from build123d import *

# Parameters (mm, degrees)
BOSS_EXTRUDE1_DEPTH = 50
BOSS_EXTRUDE2_DEPTH = 140.997088


with BuildPart() as part:
    # Sketch2 → Boss-Extrude1 (new body)
    with BuildSketch(Plane.XY.offset(17)):
        with BuildLine():
            Line((70.444464788, 96.391350971), (18.723576719, 85.49867955))
            ThreePointArc((18.723576719, 85.49867955), (18.658589867, 95.297259441), (14.88570491, 86.253934263))
            Line((14.88570491, 86.253934263), (-14.993863644, 86.253934263))
            ThreePointArc((-14.993863644, 86.253934263), (-18.766748601, 95.297259441), (-18.831735453, 85.49867955))
            Line((-18.831735453, 85.49867955), (-70.552623522, 96.391350971))
            Line((-70.552623522, 96.391350971), (-70.552623522, 101.391350971))
            Line((-70.552623522, 101.391350971), (70.444464788, 101.391350971))
            Line((70.444464788, 101.391350971), (70.444464788, 96.391350971))
        make_face()
    extrude(amount=-BOSS_EXTRUDE1_DEPTH)

    # Sketch7 → Boss-Extrude2 (add)
    with BuildSketch(Plane.ZY.offset(70.552623522)):
        Polygon((17, 131.391350971), (2, 131.391350971), (-33, 101.391350971), (17, 101.391350971), align=None)
    extrude(amount=-BOSS_EXTRUDE2_DEPTH)


solid = part.part
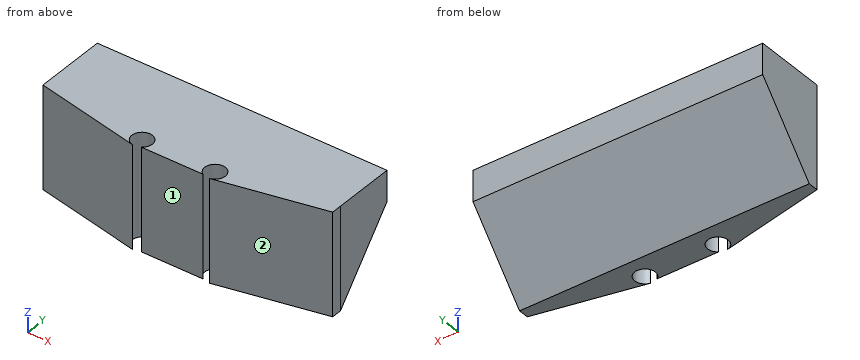
CAD build for the part. Positions are in the model's coordinates, mm. Face numbers are marked on the shaded views. A direction names the side the tool comes from. Round coordinates to 2 decimals unless told otherwise and drop trailing zeros. Loops run counter-clockwise (first coordinate to the right, second up) from the corner with the lowest first, then second, coordinate; pieces in that order, holes last.
(1) Which spindle directions (+Z, -Z, +X, -X, +Y, -Y) get a long thin tool onto all of the face, cutting with end or side? Do the marked faces 1 and 2. Say none if no direction does.
(2) Cut at A-A (y = 92.5). Give the cut face in (x, z).
(3) Cut at B-B (x = 0.5). Give the cut face in (y, z), plus the area to 3 significant figures.
(4) Cut at C-C (z = -16). Give the cut face in (x, y), plus the area to 3 significant figures.
(5) Drop flat-ended pins along their axis: pin 1 (4 mm diameter, centred on x = -9, z = -7, fed in from +Y); pin 2 (2 mm diameter, centred on x = -41, z = -18.5, fed in from +Y); pin 3 (5 mm diameter, centred on x = -37, z = -2.5, fed in from -Y). Give the stop position or say it passes through.
(6) Cut at D-D (y = 110.5). Give the cut face in (x, z).
(7) Wall check: line 1 along Y through (x, z) = (22, -23); line 2 along Y through (x, z) = (-34, 2); line 3 along Z through (x, y) = (19, 101.5). Give the ranges that are in metal, low to high.
Findings below:
1. face 1: +Z, -Z, -Y
1. face 2: +Z, -Z, +X, -Y
2. outline: (-52.08, -33) - (-22.33, -33) - (-22.33, 17) - (-52.08, 17) - close; (-13.27, -33) - (13.16, -33) - (13.16, 17) - (-13.27, 17) - close; (22.23, -33) - (51.97, -33) - (51.97, 17) - (22.23, 17) - close
3. outline: (86.25, -33) - (101.39, -33) - (131.39, 2) - (131.39, 17) - (86.25, 17) - close
3. area: 1,730 mm2
4. outline: (-70.55, 96.39) - (-18.83, 85.5) arc R5 cw (long way) to (-14.99, 86.25) - (14.89, 86.25) arc R5 cw (long way) to (18.72, 85.5) - (70.44, 96.39) - (70.44, 115.96) - (-70.55, 115.96) - close
4. area: 3,550 mm2
5. pin 1: stops at y = 125.39
5. pin 2: stops at y = 114.68
5. pin 3: stops at y = 88.8
6. outline: (-70.55, -22.37) - (70.44, -22.37) - (70.44, 17) - (-70.55, 17) - close
7. line 1: y = 86.19 to 87.85, 92.93 to 109.96
7. line 2: y = 88.69 to 131.39
7. line 3: z = -32.87 to 17
